Answer from the drawing. Dimensions are ordinates in mm from the lowest x, y and z of the part. Round coordinates to 2 decimals unless told otherwise and drop trailing zeros. Order: outer loops, then holes, each group sorted by start corner. A loop starts at its lowest first (then second) coordinate and runs counter-clockwise, first axis right, second up. Notation, with made-up numbers: M 55.5,-4.75 L 101.5,-4.75 A22 cw 101.5,12.25 Z; hole C 67,-2 d7. An arc over 180 degrees is marked long. Answer as a JSON object with one key per item and string values. Group by question number.
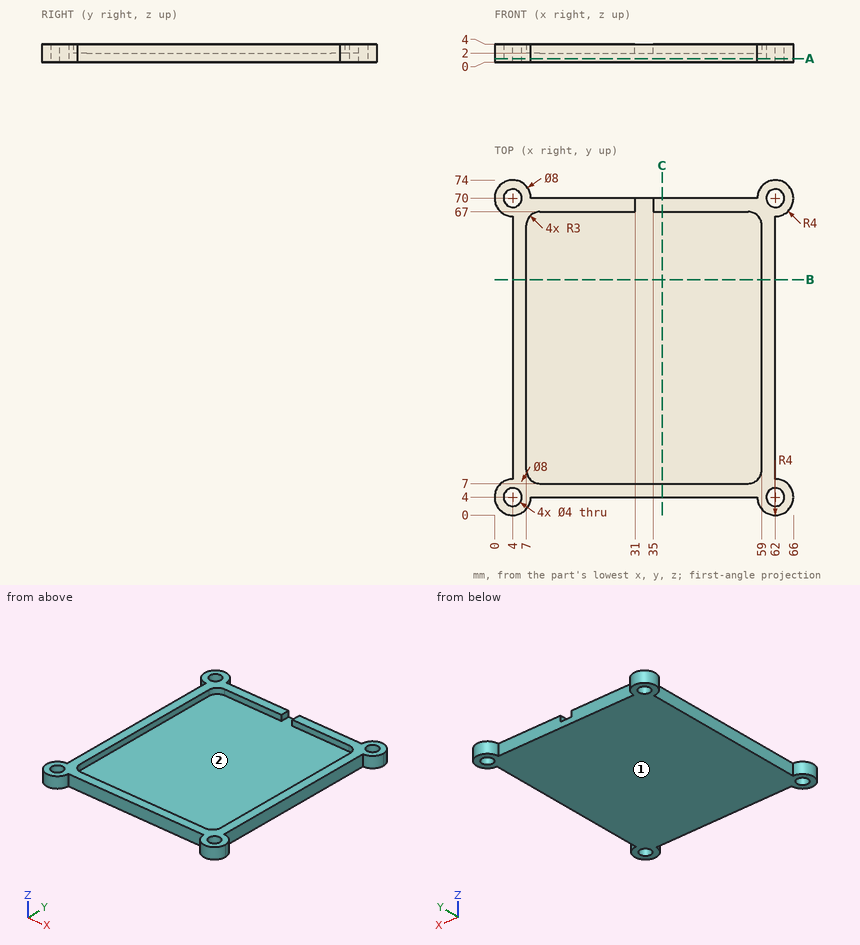
Item 1: Each of these flat-tipped pins is pushed along its axis until it touches: pin 1 (1 mm diameter, centred on y = 11, z = 1, fed in from -X); pin 2 (1 mm diameter, centred on x = 47.5, z = 3, fed in from -Y); pin 3 (1.2 mm diameter, centred on y = 38, z = 1.5, fed in from +X); pin 4 (2.5 mm diameter, centred on x = 62, y = 4, fed in from +Z). Where does it stop, or does it pass through?
Item 2: The mould has two halves that part along Y. Classify the marked faces 1 and 2: +Y half, -Y half, draft (parallel to the pull), parting line (faces both ways), or undercut.
Item 3: Consider L1, parallel to X at y = 45, z = 3.55; L2, parallel to Y at x = 5, z = 2.05; L3, parallel to X at y = 31.5, z = 1.2. Determine where each line is inside the solid, lowest interval first.
Item 4: Find section C-C (x = 37). Give the vertices of the cut face in (y, z).
Item 5: Find section B-B (y = 52). Give the vertices of the cut face in (x, z).
Item 6: Find section A-A (z = 0.75). Give the vertices of the cut face in (x, y).
Responses:
{
 "1": {"pin 1": "stops at x = 4", "pin 2": "stops at y = 4", "pin 3": "stops at x = 62", "pin 4": "passes through"},
 "2": {"face 1": "draft", "face 2": "undercut"},
 "3": {"L1": "x = 4 to 7, 59 to 62", "L2": "y = 0.13 to 2.27, 5.73 to 68.27, 71.73 to 73.87", "L3": "x = 4 to 62"},
 "4": {"outline": "M 4,0 L 70,0 L 70,4 L 67,4 L 67,2 L 7,2 L 7,4 L 4,4 Z"},
 "5": {"outline": "M 4,0 L 62,0 L 62,4 L 59,4 L 59,2 L 7,2 L 7,4 L 4,4 Z"},
 "6": {"outline": "M 4,8 A4 ccw long 8,4 L 58,4 A4 ccw long 62,8 L 62,66 A4 ccw long 58,70 L 8,70 A4 ccw long 4,66 Z; hole C 4,4 d4; hole C 4,70 d4; hole C 62,4 d4; hole C 62,70 d4"}
}
